Source: CAD feature listing. Evaluate the final solid. Frame: model axes, mm. Face numbers are marked on the shaded views. A direction names the side the tool comes from. Give positions to 0.01 mm unless a question says otherwise; leave off trailing zeros. Loops run counter-clockwise (first coordinate to the right, second up) from the corner with the lowest first, then second, coordinate; pieces in that order, holes last. Notation, with made-up numbers: (44.5, 31) - (97.5, 31) arc R23 ccw to (97.5, 42) - close; hole circle Ø11 at (-15.75, 77). An arc over 180 degrees is marked (long way). Put each result on its own line as item: value.
```python
from build123d import *

# Parameters (mm, degrees)
ESQUISSE1_R             = 32.5
BOSS_EXTRU_1_DEPTH      = 20
ESQUISSE2_R             = 27.5
BOSS_EXTRU_2_DEPTH      = 80
ESQUISSE3_R             = 16.05
ENL_V_MAT_EXTRU_1_DEPTH = 81


with BuildPart() as part:
    # Esquisse1 → Boss.-Extru.1 (new body)
    with BuildSketch(Plane.XY):
        Circle(ESQUISSE1_R)
    extrude(amount=BOSS_EXTRU_1_DEPTH)

    # Esquisse2 → Boss.-Extru.2 (add)
    with BuildSketch(Plane.XY):
        Circle(ESQUISSE2_R)
    extrude(amount=BOSS_EXTRU_2_DEPTH)

    # Esquisse3 → Enlèv. mat.-Extru.1 (cut, through all)
    with BuildSketch(Plane(origin=(0, 0, 0), x_dir=(-1, 0, 0), z_dir=(0, 0, -1))):
        Circle(ESQUISSE3_R)
    extrude(amount=-ENL_V_MAT_EXTRU_1_DEPTH, mode=Mode.SUBTRACT)


solid = part.part
```
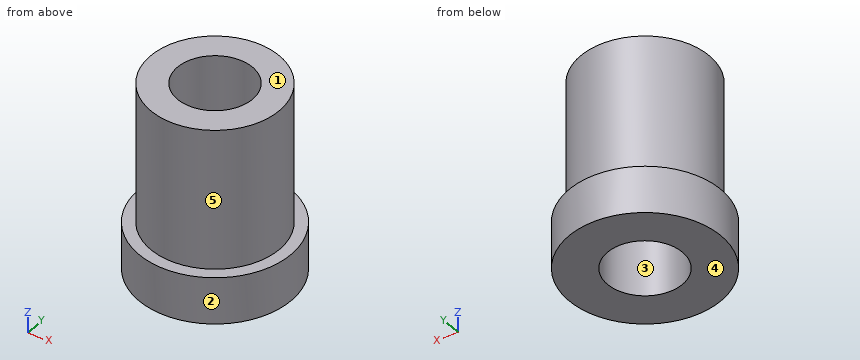
1) Material intervals for line 1 along Y through (x, z) = (0, 46); line 2 along Z through (x, y) = (-21, -19.5); line 3 along X through (y, z) = (-2.5, 38), sorted ascending. Write a range as [from, to].
Check result:
line 1: [-27.5, -16.05], [16.05, 27.5]
line 2: [0, 20]
line 3: [-27.39, -15.85], [15.85, 27.39]
2) Section query C-C, the plane z = 12. Output: boundary loops of the cut face in (x, y).
Check result:
outline: circle Ø65 at (0, 0); hole circle Ø32.1 at (0, 0)
3) Section query A-A, the plane x = 0. Output: boundary loops of the cut face in (y, z), plus the area to 3 significant figures.
Check result:
outline: (-32.5, 0) - (-16.05, 0) - (-16.05, 80) - (-27.5, 80) - (-27.5, 20) - (-32.5, 20) - close; (16.05, 0) - (32.5, 0) - (32.5, 20) - (27.5, 20) - (27.5, 80) - (16.05, 80) - close
area: 2,030 mm²
4) Section query D-D, the plane y = -22. Output: boundary loops of the cut face in (x, z).
Check result:
outline: (-23.92, 0) - (23.92, 0) - (23.92, 20) - (16.5, 20) - (16.5, 80) - (-16.5, 80) - (-16.5, 20) - (-23.92, 20) - close
5) Access query for the marked faces 4 and 5. Directions: +Z, -Z, +X, -X, +Y, -Y. A direction counts if a zero-diameter tool reaches every point of the face in a straight line with its end or side. Return the directions, or none.
Check result:
face 4: -Z, +X, -X, +Y, -Y
face 5: +Z
6) Pin query (flat end, axial travel): P1, Ø3, axis at x = -16.5, z = 51.5, coming from the -Y side; P2, Ø10, axis at y = 21, z = 32, coming from the +X side; P3, Ø8, axis at y = 4.5, z = 41, coming from the +X side. Return the tip coordinate at first contact, or that it passes through.
Check result:
P1: y = -23.05
P2: x = 22.37
P3: x = 27.5
7) Mould query, pull axis X, two halves, no side actions, for the marked faces 1, 2 and 3. Classes: pulls with the +X half, pulls with the -X half, needs draft (parallel to the pull), parting line crosses it, or undercut.
Check result:
face 1: needs draft
face 2: parting line crosses it
face 3: undercut
